Source: CAD feature listing. Evaluate the final solid. Frame: model axes, mm. A direction names the side the tool comes from. Give positions to 0.01 mm unless a question says otherwise; leave off trailing zeros. Order: outer loops, then holes, each group sorted by start corner. A loop starts at its lowest first (then second) coordinate and runs counter-clockwise, first axis right, second up. Notation, with made-up numbers: M 62,-34.5 L 100,-34.5 A30 cw 100,4.5 Z; hole C 4,83 d10. An arc over 180 degrees is marked long. Use CSV: the item, a comma, the result in double quotes. Start each with the question number.
Item 1: Ray query, probe 1 along X at (y, z) = (1.7, 13); probe 2 along X at (y, z) = (2.3, 13.5); probe 3 along Z at (x, y) = (24.5, 1.65). Return the intervals inside material, ascending. Write a range as from..to.
Item 2: Section query C-C on x = 12. Return loops of the section in (y, z).
Item 3: Section query A-A on z = 21.5. Return loops of the section in (x, y).
Item 4: Pull-direction query (X, two-part tool) for faces 4 (the face through (12.51, 2.03, 12.45)), 5 (the face through (32, 2, 25)), 6 (the face through (4, 2, 12)); classes: +X half, -X half, draft (parallel to the pull), parting line (faces both ways), or undercut.
Item 5: Section query D-D on x = 30. Return loops of the section in (y, z), and give its area (3 significant figures).
Item 6: First-contact query: pin 1 (1.2 mm diameter, centred on x = 29.5, y = 1.5, fed in from -Z); pin 2 (1.2 mm diameter, centred on x = 19.5, y = 1.5, fed in from +Z). Flat tips, straight axial feed; report the tip coordinate or a pass-through.
Item 7: Access query for faces 1 (the face through (2, 2, 17.5)), 2 (the face through (26, 2, 7)), 3 (the face through (21, 2, 21)). Directions: +Z, -Z, +X, -X, +Y, -Y. A direction counts if a zero-diameter tool reaches every point of the face in a straight line with its end or side. Return the directions, or none.
Item 8: Section query B-B on y = 0.5. Return loops of the section in (x, z), and give its area (3 significant figures).
from build123d import *

# Parameters (mm, degrees)
SKETCH1_W           = 38
SKETCH1_H           = 25
BOSS_EXTRUDE1_DEPTH = 4
SKETCH2_W           = 24
SKETCH2_H           = 7
CUT_EXTRUDE1_DEPTH  = 46.661800227
SKETCH3_W           = 4
SKETCH3_H           = 10
CUT_EXTRUDE2_DEPTH  = 46.661800227
SKETCH4_W           = 10
SKETCH4_H           = 4
CUT_EXTRUDE3_DEPTH  = 46.661800227
SKETCH5_R           = 0.75
CUT_EXTRUDE4_DEPTH  = 46.661800227


with BuildPart() as part:
    # Sketch1 → Boss-Extrude1 (new body)
    with BuildSketch(Plane(origin=(0, 0, 0), x_dir=(1, 0, 0), z_dir=(0, 1, 0))):
        with Locations((19, -12.5)):
            Rectangle(SKETCH1_W, SKETCH1_H)
    extrude(amount=BOSS_EXTRUDE1_DEPTH)

    # Sketch2 → Cut-Extrude1 (cut, through all)
    with BuildSketch(Plane(origin=(0, 4, 0), x_dir=(1, 0, 0), z_dir=(0, 1, 0))):
        with Locations((26, -3.5)):
            Rectangle(SKETCH2_W, SKETCH2_H)
    extrude(amount=-CUT_EXTRUDE1_DEPTH, mode=Mode.SUBTRACT)

    # Sketch3 → Cut-Extrude2 (cut, through all)
    with BuildSketch(Plane.XZ):
        with Locations((2, 12.5)):
            Rectangle(SKETCH3_W, SKETCH3_H)
    extrude(amount=-CUT_EXTRUDE2_DEPTH, mode=Mode.SUBTRACT)

    # Sketch4 → Cut-Extrude3 (cut, through all)
    with BuildSketch(Plane(origin=(0, 0, 0), x_dir=(-1, 0, 0), z_dir=(0, -1, 0))):
        with Locations((-21, -23)):
            Rectangle(SKETCH4_W, SKETCH4_H)
    extrude(amount=-CUT_EXTRUDE3_DEPTH, mode=Mode.SUBTRACT)

    # Sketch5 → Cut-Extrude4 (cut, through all)
    with BuildSketch(Plane(origin=(0, 4, 0), x_dir=(1, 0, 0), z_dir=(0, 1, 0))):
        with Locations(Location((12, -13, 0), (0, 0, 270))):
            Circle(SKETCH5_R)
    extrude(amount=-CUT_EXTRUDE4_DEPTH, mode=Mode.SUBTRACT)


solid = part.part
Verdict:
1,probe 1,"4..11.25, 12.75..38"
1,probe 2,"4..11.44, 12.56..38"
1,probe 3,"7..21"
2,outline,"M 0,0 L 4,0 L 4,12.25 L 0,12.25 Z; M 0,13.75 L 4,13.75 L 4,25 L 0,25 Z"
3,outline,"M 0,0 L 16,0 L 16,4 L 0,4 Z; M 26,0 L 38,0 L 38,4 L 26,4 Z"
4,face 4,"undercut"
4,face 5,"draft"
4,face 6,"-X half"
5,outline,"M 0,7 L 4,7 L 4,25 L 0,25 Z"
5,area,"72.0 mm2"
6,pin 1,"z = 7"
6,pin 2,"z = 21"
7,face 1,"-X, +Y, -Y"
7,face 2,"-Z, +X, +Y, -Y"
7,face 3,"+Z, +Y, -Y"
8,outline,"M 0,0 L 14,0 L 14,7 L 38,7 L 38,25 L 26,25 L 26,21 L 16,21 L 16,25 L 0,25 L 0,17.5 L 4,17.5 L 4,7.5 L 0,7.5 Z; hole C 12,13 d1.5"
8,area,"700 mm2"
